from build123d import *

# Parameters (mm, degrees)
FILLET1_R   = 0.2
HEX_2_DEPTH = 1.56


with BuildPart() as part:
    # BodySke → BaseBody (revolve)
    with BuildSketch(Plane.XY):
        with BuildLine():
            Line((22.75, 0), (22.75, 2.055))
            Line((22.75, 2.055), (22.305, 2.5))
            Line((22.305, 2.5), (2.75, 2.5))
            Line((2.75, 2.5), (2.75, 4.75))
            Line((2.75, 4.75), (2.37, 4.75))
            ThreePointArc((2.37, 4.75), (0.992680215, 3.754414901), (0, 2.375))
            Line((0, 2.375), (0, 0))
            Line((0, 0), (22.75, 0))
        make_face()
    revolve(axis=Axis((0, 0, 0), (1, 0, 0)))

    # Fillet1
    fillet1_edges = [part.edges().sort_by_distance(p)[0] for p in [
        (2.75, -2.5, 0),
    ]]
    fillet(fillet1_edges, radius=FILLET1_R)

    # Sketch2 → PreBroach (revolve, cut)
    with BuildSketch(Plane.XY):
        Polygon((0, 1.5), (1.56, 1.5), (2.426025404, 0), (0, 0), align=None)
    revolve(axis=Axis((0, 0, 0), (1, 0, 0)), mode=Mode.SUBTRACT)

    # Sketch3 → Hex 2 (cut)
    with BuildSketch(Plane(origin=(0, 0, 0), x_dir=(0, 0, -1), z_dir=(1, 0, 0))):
        Polygon((-1.5, -0.866025404), (-1.5, 0.866025404), (0, 1.732050808), (1.5, 0.866025404), (1.5, -0.866025404), (0, -1.732050808), align=None)
    extrude(amount=HEX_2_DEPTH, mode=Mode.SUBTRACT)


solid = part.part
Build history of the part. All positions in model axes, mm. A direction names the side the tool comes from. Coordinates: 2 decimals unless noted, no trailing zeros. Write each loop counter-clockwise with the first axis right and the second up, starting at its lowest first coordinate (ties: lowest second). Pieces come first, ordered by that corner, then holes.
(1) Cut at A-A on x = 11. List the corners of the cut face in (y, z), and give its area (3 significant figures).
(2) Mould opens along Z. For faces 1 (the flat face through (1, 0, -1.5)), 2 (the flat face through (0.769, -1.293, -0.76)), 3 (the cylindrical face through (12.49, -0.54, -2.44)), 4 (the flat face through (0, 0, -2)) say: pulls with the +Z half, pulls with the -Z half, needs draft (parallel to the pull), parting line crosses it, or undercut.
(3) Drill centre lines: line 1 (Z direction, x = 15.75, y = -2); line 2 (X direction, y = -1, z = 4.25); line 3 (X direction, y = -3, z = 2). Where is each one in solid material? Low to high.
(4) Pin check, flat tips, straight feed: pin 1 Ø1.5 at (x, z) = (11, 3.5) entering from +Y; pin 2 Ø1.2 at (x, y) = (0.5, 0) entering from +Z; pin 3 Ø1 at (x, y) = (17, -2.5) entering from +Z; pin 4 Ø3 at (x, z) = (18, -3) entering from -Y. Stop position of each tip, or through.
(5) 3-axis set-ups, long thin cutter, end or side, ignore diameter. For faces 5 (the cylindrical face through (2.557, 2.192, -4.214)), 6 (the flat face through (2.75, -2.04, -2.04)), 7 (the flat face through (0.769, 1.305, -0.74)): which of +Z, -Z, +X, -X, +Y, -Y reach the whole face in a straight line?
(6) Cut at B-B on y = -4. List the corners of the cut face in (x, z).
Working result:
1. outline: circle Ø5 at (0, 0)
1. area: 19.6 mm2
2. face 1: undercut
2. face 2: undercut
2. face 3: parting line crosses it
2. face 4: needs draft
3. line 1: z = -1.5 to 1.5
3. line 2: x = 1.72 to 2.75
3. line 3: x = 0.85 to 2.75
4. pin 1: passes through
4. pin 2: stops at z = 3.86
4. pin 3: stops at z = 1.5
4. pin 4: stops at y = -2
5. face 5: +X, -X
5. face 6: +X
5. face 7: -X
6. outline: (2.37, -2.56) - (2.75, -2.56) - (2.75, 2.56) - (2.37, 2.56) arc R3.5 ccw to start
